Design review of the part built by this model. Coordinates are the model's own, in mm. Face numbers are marked on the shaded views. A direction names the side the tool comes from. Round coordinates to 2 decimals unless told otherwise and drop trailing zeros. Loops run counter-clockwise (first coordinate to the right, second up) from the corner with the lowest first, then second, coordinate; pieces in that order, holes last. Notation, with made-up numbers: (78, 55.5) -> (131, 55.5) arc R24 cw to (131, 82.5) -> close; hole circle Ø1 at (-24.5, 40.25). An arc over 180 degrees is marked (long way). Use a Markdown table: item, result. Add a question column.
from build123d import *

# Parameters (mm, degrees)
F1_DEPTH = 5.08
F2_DEPTH = 7.62
F3_R     = 1.27


with BuildPart() as f1:
    # F0 (on Top) → F1 (new body)
    with BuildSketch(Plane.XY):
        with BuildLine():
            ThreePointArc((4.6933080252, -1.9440318364), (4.9823892244, -0.9910588358), (5.08, 0))
            Line((5.08, 0), (3.81, 0))
            ThreePointArc((3.81, 0), (3.7367919183, 0.7432941269), (3.5199810189, 1.4580238773))
            Line((3.5199810189, 1.4580238773), (4.6933080252, 1.9440318364))
            ThreePointArc((4.6933080252, 1.9440318364), (4.2238656305, 2.8222967837), (3.5921024484, 3.5921024484))
            Line((3.5921024484, 3.5921024484), (2.6940768363, 2.6940768363))
            ThreePointArc((2.6940768363, 2.6940768363), (2.1167225878, 3.1678992229), (1.4580238773, 3.5199810189))
            Line((1.4580238773, 3.5199810189), (1.9440318364, 4.6933080252))
            ThreePointArc((1.9440318364, 4.6933080252), (0.9910588358, 4.9823892244), (0, 5.08))
            Line((0, 5.08), (0, 3.81))
            ThreePointArc((0, 3.81), (-0.7432941269, 3.7367919183), (-1.4580238773, 3.5199810189))
            Line((-1.4580238773, 3.5199810189), (-1.9440318364, 4.6933080252))
            ThreePointArc((-1.9440318364, 4.6933080252), (-2.8222967837, 4.2238656305), (-3.5921024484, 3.5921024484))
            Line((-3.5921024484, 3.5921024484), (-2.6940768363, 2.6940768363))
            ThreePointArc((-2.6940768363, 2.6940768363), (-3.1678992229, 2.1167225878), (-3.5199810189, 1.4580238773))
            Line((-3.5199810189, 1.4580238773), (-4.6933080252, 1.9440318364))
            ThreePointArc((-4.6933080252, 1.9440318364), (-4.9823892244, 0.9910588358), (-5.08, 0))
            Line((-5.08, 0), (-3.81, 0))
            ThreePointArc((-3.81, 0), (-3.7367919183, -0.7432941269), (-3.5199810189, -1.4580238773))
            Line((-3.5199810189, -1.4580238773), (-4.6933080252, -1.9440318364))
            ThreePointArc((-4.6933080252, -1.9440318364), (-4.2238656305, -2.8222967837), (-3.5921024484, -3.5921024484))
            Line((-3.5921024484, -3.5921024484), (-2.6940768363, -2.6940768363))
            ThreePointArc((-2.6940768363, -2.6940768363), (-2.1167225878, -3.1678992229), (-1.4580238773, -3.5199810189))
            Line((-1.4580238773, -3.5199810189), (-1.9440318364, -4.6933080252))
            ThreePointArc((-1.9440318364, -4.6933080252), (-0.9910588358, -4.9823892244), (0, -5.08))
            Line((0, -5.08), (0, -3.81))
            ThreePointArc((0, -3.81), (0.7432941269, -3.7367919183), (1.4580238773, -3.5199810189))
            Line((1.4580238773, -3.5199810189), (1.9440318364, -4.6933080252))
            ThreePointArc((1.9440318364, -4.6933080252), (2.8222967837, -4.2238656305), (3.5921024484, -3.5921024484))
            Line((3.5921024484, -3.5921024484), (2.6940768363, -2.6940768363))
            ThreePointArc((2.6940768363, -2.6940768363), (3.1678992229, -2.1167225878), (3.5199810189, -1.4580238773))
            Line((3.5199810189, -1.4580238773), (4.6933080252, -1.9440318364))
        make_face()
    extrude(amount=F1_DEPTH)

    # F0 (on Top) → F2 (join)
    with BuildSketch(Plane.XY):
        with BuildLine():
            Line((0, 3.81), (0, 5.08))
            ThreePointArc((0, 5.08), (-0.9910588358, 4.9823892244), (-1.9440318364, 4.6933080252))
            Line((-1.9440318364, 4.6933080252), (-1.4580238773, 3.5199810189))
            ThreePointArc((-1.4580238773, 3.5199810189), (-0.7432941269, 3.7367919183), (0, 3.81))
        make_face()
        with BuildLine():
            Line((2.6940768363, 2.6940768363), (3.5921024484, 3.5921024484))
            ThreePointArc((3.5921024484, 3.5921024484), (2.8222967837, 4.2238656305), (1.9440318364, 4.6933080252))
            Line((1.9440318364, 4.6933080252), (1.4580238773, 3.5199810189))
            ThreePointArc((1.4580238773, 3.5199810189), (2.1167225878, 3.1678992229), (2.6940768363, 2.6940768363))
        make_face()
        with BuildLine():
            Line((3.81, 0), (5.08, 0))
            ThreePointArc((5.08, 0), (4.9823892244, 0.9910588358), (4.6933080252, 1.9440318364))
            Line((4.6933080252, 1.9440318364), (3.5199810189, 1.4580238773))
            ThreePointArc((3.5199810189, 1.4580238773), (3.7367919183, 0.7432941269), (3.81, 0))
        make_face()
        with BuildLine():
            Line((-2.6940768363, 2.6940768363), (-3.5921024484, 3.5921024484))
            ThreePointArc((-3.5921024484, 3.5921024484), (-4.2238656305, 2.8222967837), (-4.6933080252, 1.9440318364))
            Line((-4.6933080252, 1.9440318364), (-3.5199810189, 1.4580238773))
            ThreePointArc((-3.5199810189, 1.4580238773), (-3.1678992229, 2.1167225878), (-2.6940768363, 2.6940768363))
        make_face()
        with BuildLine():
            ThreePointArc((-5.08, 0), (-4.9823892244, -0.9910588358), (-4.6933080252, -1.9440318364))
            Line((-4.6933080252, -1.9440318364), (-3.5199810189, -1.4580238773))
            ThreePointArc((-3.5199810189, -1.4580238773), (-3.7367919183, -0.7432941269), (-3.81, 0))
            Line((-3.81, 0), (-5.08, 0))
        make_face()
        with BuildLine():
            ThreePointArc((-3.5921024484, -3.5921024484), (-2.8222967837, -4.2238656305), (-1.9440318364, -4.6933080252))
            Line((-1.9440318364, -4.6933080252), (-1.4580238773, -3.5199810189))
            ThreePointArc((-1.4580238773, -3.5199810189), (-2.1167225878, -3.1678992229), (-2.6940768363, -2.6940768363))
            Line((-2.6940768363, -2.6940768363), (-3.5921024484, -3.5921024484))
        make_face()
        with BuildLine():
            ThreePointArc((0, -5.08), (0.9910588358, -4.9823892244), (1.9440318364, -4.6933080252))
            Line((1.9440318364, -4.6933080252), (1.4580238773, -3.5199810189))
            ThreePointArc((1.4580238773, -3.5199810189), (0.7432941269, -3.7367919183), (0, -3.81))
            Line((0, -3.81), (0, -5.08))
        make_face()
        with BuildLine():
            ThreePointArc((3.5921024484, -3.5921024484), (4.2238656305, -2.8222967837), (4.6933080252, -1.9440318364))
            Line((4.6933080252, -1.9440318364), (3.5199810189, -1.4580238773))
            ThreePointArc((3.5199810189, -1.4580238773), (3.1678992229, -2.1167225878), (2.6940768363, -2.6940768363))
            Line((2.6940768363, -2.6940768363), (3.5921024484, -3.5921024484))
        make_face()
    extrude(amount=F2_DEPTH)

    # F3
    f3_edges = [f1.edges().sort_by_distance(p)[0] for p in [
        (-1.944032, -4.693308, 0),
    ]]
    fillet(f3_edges, radius=F3_R)


solid = f1.part
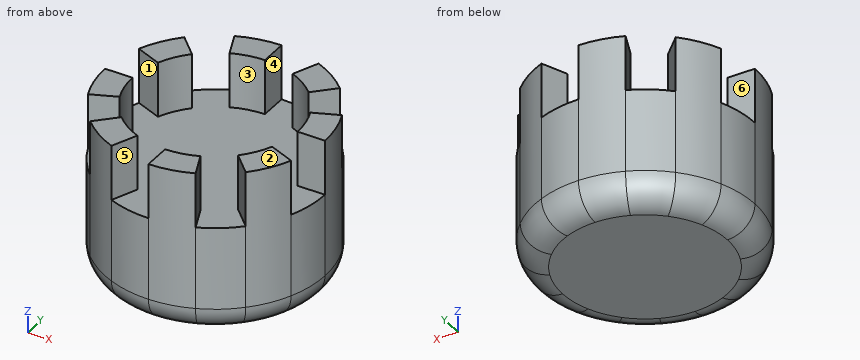
1. Consider section B-B on z = 4. State the section outline as (x, y) points.
2. Consider section C-C on z = 1. State the section outline as (x, y) points.
3. Consider section A-A on z = 6.75. Give the number of separate pieces and of enclosed holes in the cut face, plus the area to 3 significant figures.
4. For the marked faces 4, 5 and 6, list the 3-axis set-ups (+Z, -Z, +X, -X, +Y, -Y) from which the entire face can be reached by the end or side of a thin tool; tool diameter is ignored.
5. To check wall thickness, follow probe 1 along Z at (x, y) = (0.5, 1.5); probe 2 along Y at (x, z) = (-3.75, 1.75); probe 3 along Y at (x, z) = (-2.5, 3.75). State the ranges of each line that lie inside material, in increasing order. Write a range as from..to.
6. Mouldability with a two-part tool opening along Y and no side actions: class the marked faces 1, 2 and 3 as +Y half, -Y half, draft (parallel to the pull), parting line (faces both ways), or undercut.
7. Insertion check: P1, Ø1.4, axis at y = -4.5, z = 6.5, coming from the -X side; P2, Ø1.5, axis at y = 4, z = 6, coming from the +X side; P3, Ø0.6, axis at x = -4.5, z = 7, coming from the +Y side. Each pin has a flat end and moves straight along its axis. Give the tip position at first contact, or say it passes through.
Verdict:
| question | item | result |
|---|---|---|
| 1 | outline | circle Ø10.16 at (0, 0) |
| 2 | outline | circle Ø10.1 at (0, 0) |
| 3 | separate pieces | 8 |
| 3 | enclosed holes | 0 |
| 3 | area | 17.7 mm² |
| 4 | face 4 | +Z, +Y |
| 4 | face 5 | +Z, -Y |
| 4 | face 6 | +Z, -X |
| 5 | probe 1 | z = 0..5.08 |
| 5 | probe 2 | y = -3.43..3.43 |
| 5 | probe 3 | y = -4.42..4.42 |
| 6 | face 1 | undercut |
| 6 | face 2 | draft |
| 6 | face 3 | -Y half |
| 7 | P1 | stops at x = -3.37 |
| 7 | P2 | stops at x = 3.59 |
| 7 | P3 | stops at y = 2.86 |
